Read the model definition and answer for the solid it produces. Units are mm, in the model's axes. Face numbers are marked on the shaded views. Coordinates: 2 decimals unless noted, no trailing zeros. Write each loop counter-clockwise with the first axis right and the second up, starting at its lowest first coordinate (ties: lowest second). Pieces come first, ordered by that corner, then holes. Notation, with made-up numbers: (-35, 25.5) -> (-2, 25.5) arc R23 ccw to (-2, 51.5) -> close; hole circle Ø3 at (-33.75, 44.5). An arc over 180 degrees is marked (long way). Write item = value, one per line. Start each with the question number.
1) Section A-A (x = -31.25) is taken. Determine the outline of the cut face in (y, z).
2) Section B-B (z = 21) is taken. Determine the outline of the cut face in (x, y).
3) Section D-D (x = 13) is taken. Determine the outline of the cut face in (y, z).
4) Section C-C (y = 0) is taken. Determine the outline of the cut face in (x, z).
5) Find the intervals of material crossed by line 1 along X through (y, z) = (0, 24.5); line 2 along X through (y, z) = (6.5, 8.5); line 3 along Y through (x, z) = (31, 13), in increasing order. Write a range as from..to.
6) Flat-ended cylindrical pins translate along their axes: pin 1 Ø17 at (x, y) = (5, -5) entering from +Z; pin 2 Ø5 at (x, z) = (26.5, 18.5) entering from -Y; pin 3 Ø10 at (y, z) = (6.5, 5) entering from -X. Find the tip coordinate at first contact, or state that the pin passes through.
7) For a pull along X with two mould halves and no side action, classify the marked faces 1 and 2 as released by +X, released by -X, zero draft, split by the parting line, or undercut.
from build123d import *

# Parameters (mm, degrees)
F1_DEPTH = 31
F2_R     = 14.3
F2_R_2   = 10
F3_DEPTH = 31.001
F4_W     = 33
F4_H     = 80
F5_DEPTH = 21
F7_START = 10
F6_R     = 22.5
F6_R_2   = 13
F7_DEPTH = 21.001


with BuildPart() as f1:
    # F0 (on Top) → F1 (new body)
    with BuildSketch(Plane.XY):
        with BuildLine():
            ThreePointArc((-10.1844, 13.9226612628), (-17.9705989063, 10.8562655965), (-26.2597627119, 12.0040631375))
            ThreePointArc((-26.2597627119, 12.0040631375), (-44.25, 0), (-26.2597627119, -12.0040631375))
            ThreePointArc((-26.2597627119, -12.0040631375), (-17.9705989063, -10.8562655965), (-10.1844, -13.9226612628))
            ThreePointArc((-10.1844, -13.9226612628), (-5.3570791116, -16.3970791116), (0, -17.25))
            ThreePointArc((0, -17.25), (5.3570791116, -16.3970791116), (10.1844, -13.9226612628))
            ThreePointArc((10.1844, -13.9226612628), (17.9705989063, -10.8562655965), (26.2597627119, -12.0040631375))
            ThreePointArc((26.2597627119, -12.0040631375), (44.25, 0), (26.2597627119, 12.0040631375))
            ThreePointArc((26.2597627119, 12.0040631375), (17.9705989063, 10.8562655965), (10.1844, 13.9226612628))
            ThreePointArc((10.1844, 13.9226612628), (5.3570791116, 16.3970791116), (0, 17.25))
            ThreePointArc((0, 17.25), (-5.3570791116, 16.3970791116), (-10.1844, 13.9226612628))
        make_face()
    extrude(amount=F1_DEPTH)

    # F2 (on Top) → F3 (cut, through all)
    with BuildSketch(Plane.XY):
        Circle(F2_R)
        with Locations((-31.25, 0)):
            Circle(F2_R_2)
        with Locations((31.25, 0)):
            Circle(F2_R_2)
    extrude(amount=F3_DEPTH, mode=Mode.SUBTRACT)

    # F4 (on face) → F5 (cut)
    with BuildSketch(Plane.XY.offset(31)):
        Rectangle(F4_W, F4_H)
    extrude(amount=-F5_DEPTH, mode=Mode.SUBTRACT)

    # F6 (on Top) → F7 (cut)
    with BuildSketch(Plane.XY.offset(F7_START)):
        with Locations((-31.25, 0)):
            Circle(F6_R)
        with Locations((-31.25, 0)):
            Circle(F6_R_2, mode=Mode.SUBTRACT)
        with Locations((31.25, 0)):
            Circle(F6_R)
        with Locations((31.25, 0)):
            Circle(F6_R_2, mode=Mode.SUBTRACT)
    extrude(amount=F7_DEPTH, mode=Mode.SUBTRACT)


solid = f1.part
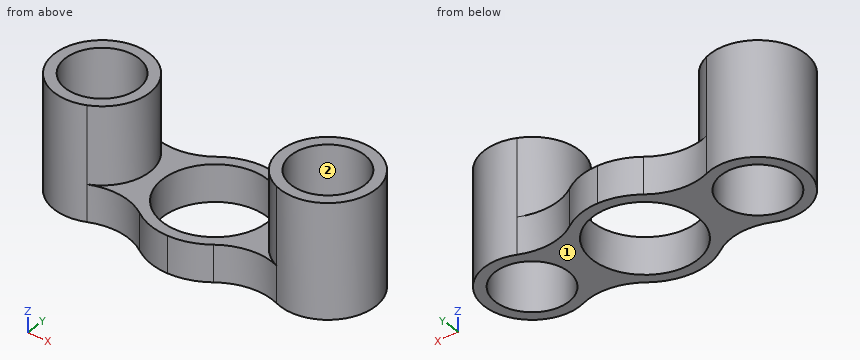
Answer key:
q1.outline = (-13, 0) -> (-10, 0) -> (-10, 31) -> (-13, 31) -> close; (10, 0) -> (13, 0) -> (13, 31) -> (10, 31) -> close
q2.outline = circle Ø26 at (-31.25, 0); circle Ø26 at (31.25, 0); hole circle Ø20 at (-31.25, 0); hole circle Ø20 at (31.25, 0)
q3.outline = (-12.26, 0) -> (-5.96, 0) -> (-5.96, 10) -> (-12.26, 10) -> close; (5.96, 0) -> (12.26, 0) -> (12.26, 10) -> (5.96, 10) -> close
q4.outline = (-44.25, 0) -> (-41.25, 0) -> (-41.25, 31) -> (-44.25, 31) -> close; (-21.25, 0) -> (-14.3, 0) -> (-14.3, 10) -> (-18.25, 10) -> (-18.25, 31) -> (-21.25, 31) -> close; (14.3, 0) -> (21.25, 0) -> (21.25, 31) -> (18.25, 31) -> (18.25, 10) -> (14.3, 10) -> close; (41.25, 0) -> (44.25, 0) -> (44.25, 31) -> (41.25, 31) -> close
q5.line_1 = -44.25..-41.25, -21.25..-18.25, 18.25..21.25, 41.25..44.25
q5.line_2 = -42.51..-38.85, -23.65..-12.74, 12.74..23.65, 38.85..42.51
q5.line_3 = -13..-10, 10..13
q6.pin_1 = 10
q6.pin_2 = -12.8
q6.pin_3 = -44.16
q7.face_1 = zero draft
q7.face_2 = undercut
